```python
from build123d import *

# Parameters (mm, degrees)
SKETCH_2_W      = 65
SKETCH_2_H      = 63
SKETCH_2_R      = 1.6
EXTRUDE_1_DEPTH = 1.5
FILLET_1_R      = 2


with BuildPart() as part:
    # 草图2 → 凸台-拉伸1 (new body)
    with BuildSketch(Plane.XY):
        Rectangle(SKETCH_2_W, SKETCH_2_H)
        with Locations((-27.5, -14)):
            Circle(SKETCH_2_R, mode=Mode.SUBTRACT)
        with Locations((-27.5, 15)):
            Circle(SKETCH_2_R, mode=Mode.SUBTRACT)
        with Locations((27.5, 15)):
            Circle(SKETCH_2_R, mode=Mode.SUBTRACT)
        with Locations((27.5, -14)):
            Circle(SKETCH_2_R, mode=Mode.SUBTRACT)
        with Locations((22.5, -26)):
            Circle(SKETCH_2_R, mode=Mode.SUBTRACT)
        with Locations((-22.5, -26)):
            Circle(SKETCH_2_R, mode=Mode.SUBTRACT)
    extrude(amount=EXTRUDE_1_DEPTH)

    # 圆角1
    fillet_1_edges = [part.edges().sort_by_distance(p)[0] for p in [
        (32.5, -31.5, 0.75),
        (-32.5, -31.5, 0.75),
        (-32.5, 31.5, 0.75),
        (32.5, 31.5, 0.75),
    ]]
    fillet(fillet_1_edges, radius=FILLET_1_R)


solid = part.part
```
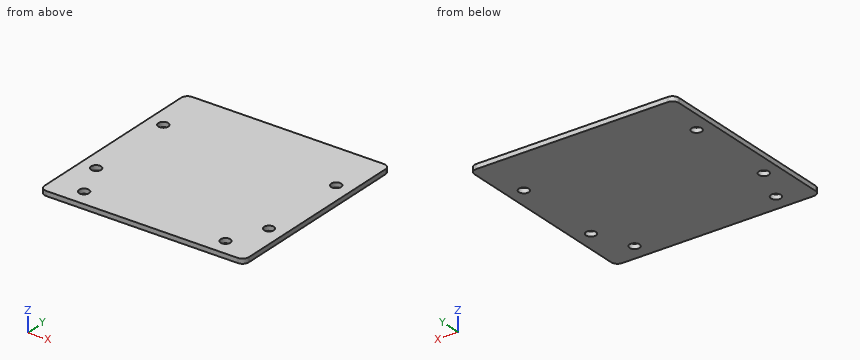
Read the model definition and answer for the solid it produces. Units are mm, in the model's axes. Coordinates: 2 decimals unless noted, no trailing zeros. Write each loop counter-clockwise with the first axis right and the second up, starting at its lowest first coordinate (ties: lowest second). Pieces come first, ordered by that corner, then holes. Notation, with made-up numbers: (85.25, -18.75) - (127.25, -18.75) arc R18 ccw to (127.25, 1.25) - close; hole circle Ø5 at (2, 6). An arc over 180 degrees is marked (long way). Answer as a JSON object with one key per item and string values. Group by question number.
1. A cutting plane is placed at A-A (x = -22.5). Determine the outline of the cut face in (y, z), plus the area to 3 significant figures.
2. A cutting plane is placed at B-B (y = -26). Determine the outline of the cut face in (x, z), plus the area to 3 significant figures.
3. This flat-tipped pin is pushed along its axis until it touches: P1, Ø3, axis at x = 22.5, y = -26, coming from the -Z side. Where does it stop, or does it pass through?
4. A cutting plane is placed at C-C (x = 27.5). Determine the outline of the cut face in (y, z).
5. Consider L1, parallel to Y at x = 27.5, z = 0.55; L2, parallel to Y at x = 28, z = 0.75; L3, parallel to Y at x = 22.5, z = 0.4. Determine where each line is inside the solid, lowest interval first. Write a range as [from, to].
Worked out:
{
 "1": {"outline": "(-31.5, 0) - (-27.6, 0) - (-27.6, 1.5) - (-31.5, 1.5) - close; (-24.4, 0) - (31.5, 0) - (31.5, 1.5) - (-24.4, 1.5) - close", "area": "89.7 mm²"},
 "2": {"outline": "(-32.5, 0) - (-24.1, 0) - (-24.1, 1.5) - (-32.5, 1.5) - close; (-20.9, 0) - (20.9, 0) - (20.9, 1.5) - (-20.9, 1.5) - close; (24.1, 0) - (32.5, 0) - (32.5, 1.5) - (24.1, 1.5) - close", "area": "87.9 mm²"},
 "3": {"P1": "passes through"},
 "4": {"outline": "(-31.5, 0) - (-15.6, 0) - (-15.6, 1.5) - (-31.5, 1.5) - close; (-12.4, 0) - (13.4, 0) - (13.4, 1.5) - (-12.4, 1.5) - close; (16.6, 0) - (31.5, 0) - (31.5, 1.5) - (16.6, 1.5) - close"},
 "5": {"L1": "y = [-31.5, -15.6], [-12.4, 13.4], [16.6, 31.5]", "L2": "y = [-31.5, -15.52], [-12.48, 13.48], [16.52, 31.5]", "L3": "y = [-31.5, -27.6], [-24.4, 31.5]"}
}
